Can you work these out from the model? Positions are in its coordinate system, mm. A direction names the side the tool comes from. Give positions to 0.01 mm unless a question says otherwise; leave off trailing zeros. Write each loop counter-clockwise with the first axis right and the second up, starting at its lowest first coordinate (ties: lowest second). Pieces come first, ordered by that corner, then holes. Notation, with made-up numbers: (-26.5, 74.25) - (13.5, 74.25) arc R28 ccw to (13.5, 93.25) - close; hole circle Ø2 at (43.25, -19). An arc over 180 degrees is marked (long way). Use a Markdown table: item, result. Add a question column.
```python
from build123d import *

# Parameters (mm, degrees)
SKETCH_1_R          = 5
EXTRUDE_1_DEPTH     = 3
EXTRUDE_3_DEPTH     = 2.5
EXTRUDE_4_DEPTH     = 2.5
EXTRUDE_START       = -8
EXTRUDE_5_DEPTH     = 2.5
SKETCH_9_R          = 2
CUT_EXTRUDE_1_DEPTH = 9


with BuildPart() as part:
    # 草图1 → 凸台-拉伸1 (new body)
    with BuildSketch(Plane(origin=(0, 0, 0), x_dir=(1, 0, 0), z_dir=(0, 1, 0))):
        Circle(SKETCH_1_R)
    extrude(amount=EXTRUDE_1_DEPTH)

    # 草图6 → 凸台-拉伸3 (add)
    with BuildSketch(Plane.XZ):
        with BuildLine():
            Line((0, -5), (0, 5))
            ThreePointArc((0, 5), (-3.535533906, 3.535533906), (-5, 0))
            Line((-5, 0), (-4.319264806, -2.518720218))
            ThreePointArc((-4.319264806, -2.518720218), (-2.490622303, -4.335527712), (0, -5))
        make_face()
        with BuildLine():
            Line((0, -18.5), (0, -5))
            ThreePointArc((0, -5), (-2.490622303, -4.335527712), (-4.319264806, -2.518720218))
            Line((-4.319264806, -2.518720218), (0, -18.5))
        make_face()
        with BuildLine():
            ThreePointArc((5, 0), (3.535533906, 3.535533906), (0, 5))
            Line((0, 5), (0, -5))
            ThreePointArc((0, -5), (2.490622303, -4.335527712), (4.319264806, -2.518720218))
            Line((4.319264806, -2.518720218), (5, 0))
        make_face()
        with BuildLine():
            ThreePointArc((4.319264806, -2.518720218), (2.490622303, -4.335527712), (0, -5))
            Line((0, -5), (0, -18.5))
            Line((0, -18.5), (4.319264806, -2.518720218))
        make_face()
    extrude_3 = extrude(amount=EXTRUDE_3_DEPTH)

    # 镜向1: 凸台-拉伸3 across plane
    add(extrude_3.mirror(Plane.ZX.offset(1.5)))

    # 草图8 → 凸台-拉伸4 (add)
    with BuildSketch(Plane(origin=(0, 5.5, 0), x_dir=(1, 0, 0), z_dir=(0, 1, 0))):
        with BuildLine():
            Line((1.25, 23.125), (0, 18.5))
            Line((0, 18.5), (-1.25, 23.125))
            Line((-1.25, 23.125), (-7.5, 0))
            ThreePointArc((-7.5, 0), (0, -7.5), (7.5, 0))
            Line((7.5, 0), (1.25, 23.125))
        make_face()
        with BuildLine():
            Line((-5, 0), (0, 18.5))
            Line((0, 18.5), (5, 0))
            ThreePointArc((5, 0), (0, -5), (-5, 0))
        make_face(mode=Mode.SUBTRACT)
        with BuildLine():
            Line((-1.25, 23.125), (0, 18.5))
            Line((0, 18.5), (1.25, 23.125))
            ThreePointArc((1.25, 23.125), (0, 23.290941974), (-1.25, 23.125))
        make_face()
    extrude(amount=-EXTRUDE_4_DEPTH)

    # 草图8<4> → 凸台-拉伸5 (add)
    with BuildSketch(Plane(origin=(0, 5.5, 0), x_dir=(1, 0, 0), z_dir=(0, 1, 0)).offset(EXTRUDE_START)):
        with BuildLine():
            Line((-7.5, 0), (-1.25, 23.125))
            ThreePointArc((-1.25, 23.125), (0, 23.290941974), (1.25, 23.125))
            Line((1.25, 23.125), (7.5, 0))
            ThreePointArc((7.5, 0), (0, -7.5), (-7.5, 0))
        make_face()
    extrude(amount=EXTRUDE_5_DEPTH)

    # 草图9 → 切除-拉伸1 (cut, through all)
    with BuildSketch(Plane.XZ.offset(2.5)):
        Circle(SKETCH_9_R)
    extrude(amount=-CUT_EXTRUDE_1_DEPTH, mode=Mode.SUBTRACT)


solid = part.part
```
Q1. Suppose I cut it at D-D (x = 6.75). Please give me the cut outline in (y, z) (3 decimals), and give its area (3 significant figures).
Q2. On a 3-axis mill with a long thin cutter (end or side, diameter ignored), from which of +Z, -Z, +X, -X, +Y, -Y can I reach the whole of each face in a straight line? I mean faces 5 (the flat face through (-4.331, 4.268, -11.724)), 6 (the flat face through (0, 3, -8)). Say none if no direction works.
Q3. Suppose I cut it at B-B (x = 0). Please give me the cut outline in (y, z).
Q4. I'm going to push flat-ended pins straight in: P1, Ø5, axis at x = 0.5, z = 1.5, coming from the +Y side; P2, Ø1, axis at x = -1.5, y = -1.5, coming from the -Z side; P3, Ø4, axis at y = 1, z = -6, coming from the +X side; P4, Ø1, axis at y = 1, z = -6, coming from the -X side. Where does each tip first touch, or does it pass through?
Q5. If we mould it in two halves opening along Z, with no side actions, what happens to faces 1 (the cylindrical face through (0, 1, -2)), 2 (the flat face through (0, 0, -8)), 3 (the cylindrical face through (-1.08, 1.48, 4.88)), 4 (the cylindrical face through (-0.16, 4.27, 7.5))? For each: released by +Z, released by -Z, zero draft, split by the parting line, or undercut.
Q6. Suppose I cut it at A-A (z = 6). Please give me the cut outline in (x, y), and give its area (3 significant figures).
Q7. Suppose I cut it at C-C (y = -1). Please give me the cut outline in (x, z) (3 decimals), and give its area (3 significant figures).
Q8. If I drill on probe 1 along Y at (x, z) = (0.5, -10.5); probe 2 along Z at (x, y) = (0, -0.5); probe 3 along Z at (x, y) = (0, 0.5), over which ranges is the centre line in solid material (lowest first)? Write a range as [from, to].
Derived:
| question | item | result |
|---|---|---|
| 1 | outline | (-2.5, -2.775) - (0, -2.775) - (0, 3.269) - (-2.5, 3.269) - close; (3, -2.775) - (5.5, -2.775) - (5.5, 3.269) - (3, 3.269) - close |
| 1 | area | 30.2 mm² |
| 2 | face 5 | -Z, -X, +Y, -Y |
| 2 | face 6 | none |
| 3 | outline | (-2.5, -23.29) - (0, -23.29) - (0, -5) - (3, -5) - (3, -23.29) - (5.5, -23.29) - (5.5, -2) - (-2.5, -2) - close; (-2.5, 2) - (5.5, 2) - (5.5, 7.5) - (3, 7.5) - (3, 5) - (0, 5) - (0, 7.5) - (-2.5, 7.5) - close |
| 4 | P1 | y = 5.5 |
| 4 | P2 | z = -23.19 |
| 4 | P3 | x = 6.35 |
| 4 | P4 | through |
| 5 | face 1 | undercut |
| 5 | face 2 | zero draft |
| 5 | face 3 | split by the parting line |
| 5 | face 4 | released by +Z |
| 6 | outline | (-4.5, -2.5) - (4.5, -2.5) - (4.5, 0) - (-4.5, 0) - close; (-4.5, 3) - (4.5, 3) - (4.5, 5.5) - (-4.5, 5.5) - close |
| 6 | area | 45.0 mm² |
| 7 | outline | (-7.5, 0) - (-1.25, -23.125) arc R4.791 ccw to (1.25, -23.125) - (7.5, 0) arc R7.5 ccw to start; hole circle Ø4 at (0, 0) |
| 7 | area | 278 mm² |
| 8 | probe 1 | [-2.5, 0], [3, 5.5] |
| 8 | probe 2 | [-23.29, -2], [2, 7.5] |
| 8 | probe 3 | [-5, -2], [2, 5] |
